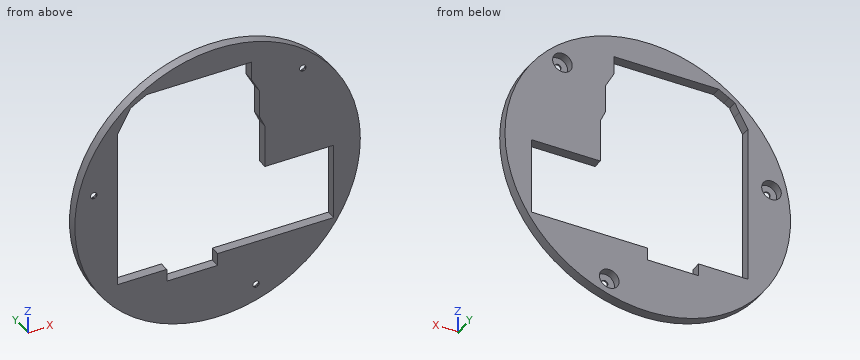
from build123d import *

# Parameters (mm, degrees)
SKETCH2_R           = 44.4
BOSS_EXTRUDE1_DEPTH = 3
CUT_EXTRUDE3_START  = 3
SKETCH3_R           = 3.05
CUT_EXTRUDE3_DEPTH  = 2.6
SKETCH4_R           = 1
CUT_EXTRUDE4_DEPTH  = 1.4


with BuildPart() as part:
    # Sketch2 → Boss-Extrude1 (new body)
    with BuildSketch(Plane(origin=(0, 0, 0), x_dir=(1, 0, 0), z_dir=(0, 1, 0))):
        with Locations((5.844668035, 0)):
            Circle(SKETCH2_R)
        Polygon((-25.306151193, 23.466427606), (-9.956472153, 23.466427606), (-9.956472153, 27.379090891), (5.844668035, 27.379090891), (5.844668035, 23.466427606), (41.936760168, 23.466427606), (41.936760168, -0.473949831), (20.582698865, -0.473949831), (20.582698865, -13.817632751), (18.922929974, -17.433557834), (18.922929974, -26.013051917), (16.376674503, -30.649762231), (16.376674503, -36.409044515), (-16.167559029, -36.409044515), (-19.414149946, -34.62617491), (-21.26171293, -33.507445335), (-22.686577877, -30.901858186), (-25.306151193, -26.111560985), align=None, mode=Mode.SUBTRACT)
    extrude(amount=BOSS_EXTRUDE1_DEPTH)

    # Sketch3 → Cut-Extrude3 (cut)
    with BuildSketch(Plane(origin=(0, 0, 0), x_dir=(1, 0, 0), z_dir=(0, 1, 0)).offset(CUT_EXTRUDE3_START)):
        with Locations((32.364967514, -29.138183119)):
            Circle(SKETCH3_R)
        with Locations((17.818925096, 37.536344625)):
            Circle(SKETCH3_R)
        with Locations((-32.649888507, -8.398161506)):
            Circle(SKETCH3_R)
    extrude(amount=-CUT_EXTRUDE3_DEPTH, mode=Mode.SUBTRACT)

    # Sketch4 → Cut-Extrude4 (cut, through all)
    with BuildSketch(Plane(origin=(0, 0.4, 0), x_dir=(1, 0, 0), z_dir=(0, 1, 0))):
        with Locations((-32.649888507, -8.398161506)):
            Circle(SKETCH4_R)
        with Locations((17.818925096, 37.536344625)):
            Circle(SKETCH4_R)
        with Locations((32.364967514, -29.138183119)):
            Circle(SKETCH4_R)
    extrude(amount=-CUT_EXTRUDE4_DEPTH, mode=Mode.SUBTRACT)


solid = part.part
Design review of the part built by this model. Coordinates are the model's own, in mm. Round coordinates to 2 decimals unless told otherwise and drop trailing zeros. Write each loop counter-clockwise with the first axis right and the second up, starting at its lowest first coordinate (ties: lowest second). Pieces come first, ordered by that corner, then holes.
Item 1: Consider section B-B on z = 16. Give the boundary of the cut face in (x, y).
Item 2: Consider section C-C on y = 2.4. Give the boundary of the cut face in (x, z).
Item 3: Consider section A-A on x = -12.5. Give the boundary of the cut face in (y, z).
Item 4: Wall thickness on L1, parallel to Z at x = 4.5, y = 2.5; L2, parallel to Z at x = 35, y = 1.2; L3, parallel to X at y = 2.75, z = 8: over which ranges is each line inside the solid? List them lowest first.
Item 5: For pin 1 Ø1.8 at (x, z) = (17.82, -37.54) entering from -Y; pin 2 Ø0.9 at (x, y) = (-1.5, 2) entering from +Z; pin 3 Ø0.9 at (y, z) = (2, -25.5) entering from -X; pin 4 Ø1.5 at (x, y) = (-14.5, 2) entering from +Z, all flat-tipped, find the tip position at first contact; note any pin that passes through.
Check values:
1. outline: (-35.57, 0) - (-25.31, 0) - (-25.31, 3) - (-35.57, 3) - close; (19.58, 0) - (47.26, 0) - (47.26, 3) - (19.58, 3) - close
2. outline: circle Ø88.8 at (5.84, 0); hole circle Ø6.1 at (-32.65, 8.4); hole (-25.31, -23.47) - (-9.96, -23.47) - (-9.96, -27.38) - (5.84, -27.38) - (5.84, -23.47) - (41.94, -23.47) - (41.94, 0.47) - (20.58, 0.47) - (20.58, 13.82) - (18.92, 17.43) - (18.92, 26.01) - (16.38, 30.65) - (16.38, 36.41) - (-16.17, 36.41) - (-19.41, 34.63) - (-21.26, 33.51) - (-25.31, 26.11) - close; hole circle Ø6.1 at (17.82, -37.54); hole circle Ø6.1 at (32.36, 29.14)
3. outline: (0, -40.43) - (3, -40.43) - (3, -23.47) - (0, -23.47) - close; (0, 36.41) - (3, 36.41) - (3, 40.43) - (0, 40.43) - close
4. L1: z = -44.38 to -27.38, 36.41 to 44.38
4. L2: z = -33.49 to -23.47, 0.47 to 27.6, 30.67 to 33.49
4. L3: x = -37.83 to -35.67, -29.63 to -25.31, 20.58 to 49.52
5. pin 1: passes through
5. pin 2: stops at z = 43.86
5. pin 3: stops at x = -30.81
5. pin 4: stops at z = 39.84
